```python
from build123d import *

# Parameters (mm, degrees)
F0_W     = 31.75
F0_H     = 31.75
F1_DEPTH = 1.5875
F0_W_2   = 6.35
F0_H_2   = 1.4605
F2_DEPTH = 1.4605
F3_R     = 1.46049
F5_DEPTH = 1.5875
F6_DEPTH = 6.35


# Not quite as in the source:
# - a fillet or chamfer is up to 0.001 mm smaller than in the source, because OpenCascade refuses the exact size
# - ends of sketch curves that miss each other by under 0.0002 mm in the source are joined


with BuildPart() as f1:
    # F0 (on Top) → F1 (new body, symmetric)
    with BuildSketch(Plane.XY):
        Polygon((17.4625, 17.4625), (-17.4625, 17.4625), (-17.4625, 1.4605), (-17.4625, 0), (-17.4625, -1.4605), (-17.4625, -17.4625), (17.4625, -17.4625), (17.4625, -1.4605), (17.4625, 0), (17.4625, 1.4605), align=None)
        Rectangle(F0_W, F0_H, mode=Mode.SUBTRACT)
        Rectangle(F0_W, F0_H)
    extrude(amount=F1_DEPTH, both=True)

    # F0 (on Top) → F2 (join, symmetric)
    with BuildSketch(Plane.XY):
        with Locations((-20.6375, 0.73025)):
            Rectangle(F0_W_2, F0_H_2)
        with Locations((-20.6375, -0.73025)):
            Rectangle(F0_W_2, F0_H_2)
        with Locations((20.6375, 0.73025)):
            Rectangle(F0_W_2, F0_H_2)
        with Locations((20.6375, -0.73025)):
            Rectangle(F0_W_2, F0_H_2)
    extrude(amount=F2_DEPTH, both=True)

    # F3 (radius 1.4605 in the source; OpenCascade refuses exactly that, so slightly less here)
    f3_edges = [f1.edges().sort_by_distance(p)[0] for p in [
        (-20.6375, -1.4605, 1.4605),
        (-20.6375, 1.4605, 1.4605),
        (-20.6375, -1.4605, -1.4605),
        (-20.6375, 1.4605, -1.4605),
        (20.6375, 1.4605, -1.4605),
        (20.6375, -1.4605, -1.4605),
        (20.6375, -1.4605, 1.4605),
        (20.6375, 1.4605, 1.4605),
    ]]
    fillet(f3_edges, radius=F3_R)

    # F4 (on face) → F5 (join)
    with BuildSketch(Plane.YZ.offset(23.8125)):
        with BuildLine():
            Line((9.525, 1.27), (0.7212287186, 1.27))
            ThreePointArc((0.7212287186, 1.27), (1.2622230895, 0.7347542799), (1.4605, 1e-05))
            ThreePointArc((1.4605, 1e-05), (1.2622230895, -0.7347542799), (0.7212287186, -1.27))
            Line((0.7212287186, -1.27), (9.525, -1.27))
            Line((9.525, -1.27), (9.525, 1.27))
        make_face()
        with BuildLine():
            Line((-0.7212287186, 1.27), (-9.525, 1.27))
            Line((-9.525, 1.27), (-9.525, -1.27))
            Line((-9.525, -1.27), (-0.7212287186, -1.27))
            ThreePointArc((-0.7212287186, -1.27), (-1.2622230895, -0.7347542799), (-1.4605, -1e-05))
            ThreePointArc((-1.4605, -1e-05), (-1.2622230895, 0.7347542799), (-0.7212287186, 1.27))
        make_face()
        with BuildLine():
            Line((0.7212287186, 1.27), (-0.7212287186, 1.27))
            ThreePointArc((-0.7212287186, 1.27), (-1.2622230895, 0.7347542799), (-1.4605, 1e-05))
            ThreePointArc((-1.4605, 1e-05), (-1.2622230895, -0.7347542799), (-0.7212287186, -1.27))
            Line((-0.7212287186, -1.27), (0.7212287186, -1.27))
            ThreePointArc((0.7212287186, -1.27), (1.2622230895, -0.7347542799), (1.4605, -1e-05))
            ThreePointArc((1.4605, -1e-05), (1.2622230895, 0.7347542799), (0.7212287186, 1.27))
        make_face()
    extrude(amount=F5_DEPTH)

    # F6 (add): a face of the model
    f6_faces = [f1.faces().sort_by_distance(p)[0] for p in [
        (0, 0, 1.5875),
    ]]
    extrude(f6_faces, amount=F6_DEPTH)


solid = f1.part
```
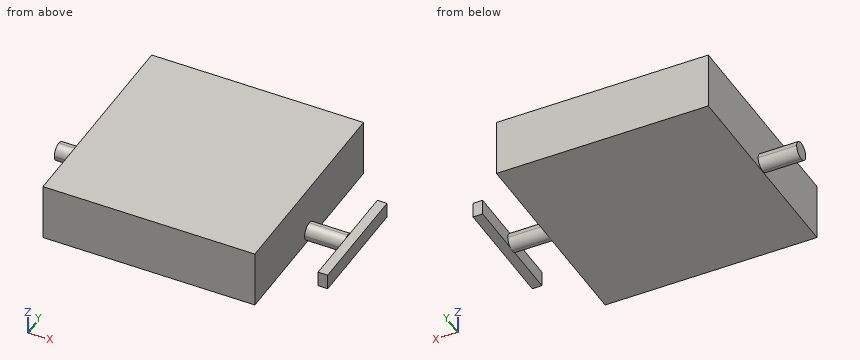
CAD build for the part. Positions are in the model's coordinates, mm. Coordinates: 2 decimals unless noted, no trailing zeros. Loops run counter-clockwise (first coordinate to the right, second up) from the corner with the lowest first, then second, coordinate; pieces in that order, holes last. Notation, with made-up numbers: (34.25, 48) - (46.25, 48) arc R21 cw to (46.25, 77) - close; hole circle Ø10 at (-20, 53). An arc over 180 degrees is marked (long way). Return JSON: item names as keys, results as strings.
1. Probe L1, parallel to Y at x = -20, z = 0; L2, parallel to X at y = -10.5, z = 6; L3, parallel to X at y = -2.5, z = -0.75. List the from-to ranges inside material, lowest first. Write a range as from..to.
Result:
{"L1": "y = -1.46..1.46", "L2": "x = -17.46..17.46", "L3": "x = -17.46..17.46, 23.81..25.4"}
2. Band-saw the part on D-D (y = 13). Give the cut face in (x, z), and give its area (3 significant figures).
Result:
{"outline": "(-17.46, -1.59) - (17.46, -1.59) - (17.46, 7.94) - (-17.46, 7.94) - close", "area": "333 mm2"}
3. Drop flat-ended pins along their axis: pin 1 (1.5 mm diameter, centred on y = -10.5, z = 3, fed in from +X); pin 2 (0.8 mm diameter, centred on y = -7, z = -0.5, fed in from -X); pin 3 (1.3 mm diameter, centred on x = 24.5, z = 0, fed in from -Y) (3 decimals). Give the stop position or say it passes through.
Result:
{"pin 1": "stops at x = 17.46", "pin 2": "stops at x = -17.46", "pin 3": "stops at y = -9.525"}
4. Band-saw the part on A-A (y = -3.5). Give the cut face in (x, z).
Result:
{"outline": "(-17.46, -1.59) - (17.46, -1.59) - (17.46, 7.94) - (-17.46, 7.94) - close; (23.81, -1.27) - (25.4, -1.27) - (25.4, 1.27) - (23.81, 1.27) - close"}
5. Band-saw the part on C-C (z = 0.5). Give the cut face in (x, y) (1 decimal).
Result:
{"outline": "(-23.8, -1.4) - (-17.5, -1.4) - (-17.5, -17.5) - (17.5, -17.5) - (17.5, -1.4) - (23.8, -1.4) - (23.8, -9.5) - (25.4, -9.5) - (25.4, 9.5) - (23.8, 9.5) - (23.8, 1.4) - (17.5, 1.4) - (17.5, 17.5) - (-17.5, 17.5) - (-17.5, 1.4) - (-23.8, 1.4) - close"}
